Design review of the part built by this model. Coordinates are the model's own, in mm. Coordinates: 2 decimals unless noted, no trailing zeros. Write each loop counter-clockwise with the first axis right and the second up, starting at its lowest first coordinate (ties: lowest second). Pieces come first, ordered by that corner, then holes. Notation, with made-up numbers: (18, 20) - (28, 20) arc R20 ccw to (28, 53) - close; hole circle Ø11 at (-1.75, 51.5). An arc over 180 degrees is marked (long way). Answer as a JSON object with one key per item and string values.
Autodesk Inventor part; units mm, degrees
ref_plane "YZ Plane" through (0, 0, 0) normal (1, 0, 0) x (0, 1, 0)
ref_plane "XZ Plane" through (0, 0, 0) normal (0, 1, 0) x (-1, 0, 0)
ref_plane "XY Plane" through (0, 0, 0) normal (0, 0, 1) x (1, 0, 0)
sketch "Boceto1" plane through (0, 0, 0) normal (0, 0, 1) x (1, 0, 0)
  line L0 (0, 0) -> (220, 0)
  line L1 (251, 0) -> (251, -25)
  line L2 (251, -25) -> (0, -25)
  line L3 (220, 0) -> (220, 85)
  line L4 (220, 85) -> (251, 85)
  line L5 (251, 85) -> (251, 0)
  line L6 (0, -25) -> (-30, -25)
  line L7 (-30, -25) -> (-30, 0)
  line L8 (-30, 0) -> (0, 0)
  dimension "d3" = 85
  dimension "d4" = 31
extrude "Extrusión1" add sketch "Boceto1" along normal blind 10
fillet "Empalme1" radius 30 1 edges at (220, 0, 5)
sketch "Boceto2" plane through (0, 0, 10) normal (0, 0, 1) x (1, 0, 0)
  line L0 (220, 30) -> (220, 85)
  line L1 (251, -25) -> (-30, -25)
  line L2 (220, 85) -> (251, 85)
  line L3 (225.1, 75) -> (239.9, 75)
  line L4 (239.9, 75) -> (239.9, 46)
  line L5 (239.9, 46) -> (225.1, 46)
  line L6 (225.1, 46) -> (225.1, 75)
  line L7 (225.1, 14) -> (239.9, 14)
  line L8 (239.9, 14) -> (239.9, -15)
  line L9 (239.9, -15) -> (225.1, -15)
  line L10 (225.1, -15) -> (225.1, 14)
  point P0 (225, 80)
  point P1 (220, 75)
  point P2 (5, -25)
  point P3 (240, -25)
  point P4 (245, -20)
  point P5 (245, 75)
  point P6 (240, 80)
  point P7 (0, 0)
  point P8 (0, -25)
  dimension "d10" = 14.8
  dimension "d11" = 14.8
  dimension "d12" = 5.1
  dimension "d14" = 10
  dimension "d15" = 29
  dimension "d16" = 29
  dimension "d17" = 10
  dimension "d82" = 5.1
extrude "Extrusión2" cut sketch "Boceto2" against normal blind 10
sketch "Boceto3" plane through (0, 0, 10) normal (0, 0, 1) x (1, 0, 0)
  line L0 (0, 0) -> (190, 0)
  line L1 (251, -25) -> (-30, -25)
  line L2 (180, -10) -> (170, -10)
  line L3 (170, -10) -> (170, -5)
  line L4 (170, -5) -> (180, -5)
  line L5 (180, -5) -> (180, -10)
  line L6 (110, -5) -> (100, -5)
  line L7 (100, -5) -> (100, -10)
  line L8 (100, -10) -> (110, -10)
  line L9 (110, -10) -> (110, -5)
  line L10 (40, -5) -> (30, -5)
  line L11 (30, -5) -> (30, -10)
  line L12 (30, -10) -> (40, -10)
  line L13 (40, -10) -> (40, -5)
  line L14 (145, -15) -> (135, -15)
  line L15 (135, -15) -> (135, -20)
  line L16 (135, -20) -> (145, -20)
  line L17 (145, -20) -> (145, -15)
  line L18 (75, -15) -> (65, -15)
  line L19 (65, -15) -> (65, -20)
  line L20 (65, -20) -> (75, -20)
  line L21 (75, -20) -> (75, -15)
  point P0 (5, 0)
  point P1 (0, -5)
  point P2 (0, -20)
  point P3 (5, -25)
  point P4 (240, -25)
  dimension "d20" = 10
  dimension "d21" = 10
  dimension "d22" = 10
  dimension "d24" = 5
  dimension "d25" = 5
  dimension "d26" = 5
  dimension "d27" = 5
  dimension "d28" = 5
  dimension "d29" = 10
  dimension "d30" = 10
  dimension "d31" = 5
  dimension "d32" = 5
  dimension "d33" = 5
  dimension "d34" = 5
  dimension "d36" = 25
  dimension "d37" = 25
  dimension "d38" = 25
  dimension "d39" = 25
extrude "Extrusión3" cut sketch "Boceto3" against normal blind 10
sketch "Boceto4" plane through (0, 0, 10) normal (0, 0, 1) x (1, 0, 0)
  line L0 (145, -15) -> (145, -20)
  line L1 (145, -20) -> (135, -20)
  line L2 (205, -20) -> (215, -20)
  line L3 (215, -20) -> (215, -15)
  line L4 (215, -15) -> (205, -15)
  line L5 (205, -15) -> (205, -20)
  point P0 (0, 0)
  dimension "d42" = 10
  dimension "d43" = 5
  dimension "d44" = 60
extrude "Extrusión4" cut sketch "Boceto4" against normal blind 10
sketch "Boceto6" plane through (0, 0, 10) normal (0, 0, 1) x (1, 0, 0)
  line L0 (237.5, 82.5) -> (227.5, 82.5)
  line L1 (227.5, 82.5) -> (227.5, 77.5)
  line L2 (227.5, 77.5) -> (237.5, 77.5)
  line L3 (237.5, 77.5) -> (237.5, 82.5)
  circle A0 centre (245.5, -17.5) radius 1.6
  circle A1 centre (245.5, 27.5) radius 1.6
  circle A2 centre (245.5, 75.9891) radius 1.6
  circle A3 centre (222.4918, 80) radius 1.6
  circle A4 centre (222.4918, 27.5) radius 1.6
  circle A5 centre (175, -17.5) radius 1.6
  circle A6 centre (166.25, -7.5) radius 1.6
  circle A7 centre (105, -17.5) radius 1.6
  circle A8 centre (70, -7.5) radius 1.6
  circle A9 centre (45, -17.5) radius 1.6
  circle A10 centre (0, -7.5) radius 1.6
  line L4 (-30, -25) -> (-30, 0)
  circle A11 centre (222.4918, -17.5) radius 1.6
  line L5 (251, 85) -> (251, -25)
  line L6 (220, 85) -> (251, 85)
  line L7 (170, -10) -> (170, -5)
  point P0 (0, 0)
  dimension "d52" = 5
  dimension "d54" = 3.2
  dimension "d55" = 3.2
  dimension "d56" = 3.2
  dimension "d57" = 3.2
  dimension "d58" = 3.2
  dimension "d60" = 3.2
  dimension "d61" = 3.2
  dimension "d62" = 3.2
  dimension "d63" = 3.2
  dimension "d64" = 3.2
  dimension "d65" = 3.2
  dimension "d80" = 30
  dimension "d81" = 3.2
  dimension "d83" = 5.5
  dimension "d84" = 5.5
  dimension "d85" = 5.5
  dimension "d92" = 2.5
  dimension "d93" = 5
  dimension "d94" = 3.75
  dimension "d95" = 75
extrude "Extrusión6" cut sketch "Boceto6" against normal blind 10
fillet "Empalme3" radius 5 1 edges at (251, -25, 5)
fillet "Empalme4" radius 5 2 edges at (-30, 0, 5) (-30, -25, 5)
fillet "Empalme5" radius 1 2 edges at (220, 85, 5) (251, 85, 5)
sketch "Boceto7" plane through (0, 0, 10) normal (0, 0, 1) x (1, 0, 0)
  line L0 (-25, 0) -> (190, 0)
  line L1 (-30, -20) -> (-30, -5)
  line L2 (-25, -5) -> (-15, -5)
  line L3 (-15, -5) -> (-15, -20)
  line L4 (-15, -20) -> (-25, -20)
  line L5 (-25, -20) -> (-25, -5)
  point P0 (0, 0)
  dimension "d74" = 10
  dimension "d75" = 15
  dimension "d76" = 5
  dimension "d77" = 5
extrude "Extrusión7" cut sketch "Boceto7" against normal blind 10
sketch "Boceto8" plane through (0, 0, 10) normal (0, 0, 1) x (1, 0, 0)
  line L0 (221, 85) -> (250, 85)
  line L1 (251, 84) -> (251, -20)
  line L2 (243, 66.5) -> (248, 66.5)
  line L3 (248, 66.5) -> (248, 56.5)
  line L4 (248, 56.5) -> (243, 56.5)
  line L5 (243, 56.5) -> (243, 66.5)
  point P0 (0, 0)
  dimension "d86" = 5
  dimension "d87" = 10
  dimension "d88" = 3
  dimension "d89" = 18.5
extrude "Extrusión8" cut sketch "Boceto8" against normal blind 10
properties part number "brazo eje z"
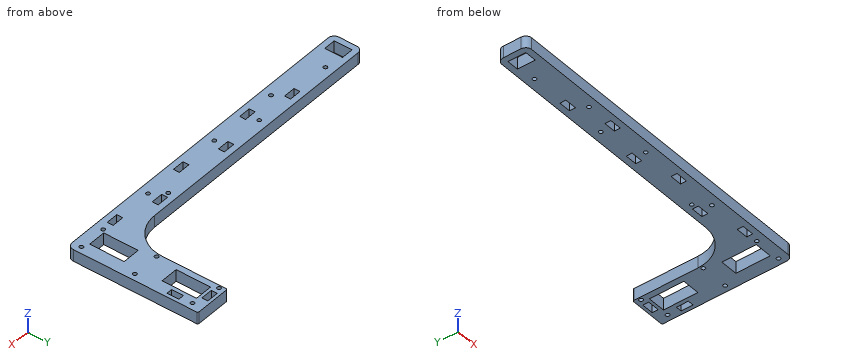
(1) Take a section at B-B, the plane x = 18.5. Write out the cut boundary in (y, z), and give its area (3 significant figures).
Solved:
{"outline": "(-25, 0) - (0, 0) - (0, 10) - (-25, 10) - close", "area": "250 mm^2"}
(2) Take a section at A-A, the plane y = 6. Write out the cut boundary in (x, z).
Solved:
{"outline": "(208, 0) - (225.1, 0) - (225.1, 10) - (208, 10) - close; (239.9, 0) - (251, 0) - (251, 10) - (239.9, 10) - close"}
(3) For pin 1 (10 mm diameter, centred on x = 3, y = -9.5, fed in from -Z); pin 2 (1.5 mm diameter, centred on y = 70, z = 2.5, fed in from -X); pin 3 (6 mm diameter, centred on y = 24, z = 8.5, fed in from -X), all flat-tipped, find the tip position at first contact; note any pin that passes through.
Solved:
{"pin 1": "stops at z = 0", "pin 2": "stops at x = 220", "pin 3": "stops at x = 218.62"}
(4) Take a section at C-C, the plane z = 3. Give the number of separate pieces and of enclosed holes in the cut face, and give its area (3 significant figures).
Solved:
{"separate pieces": "1", "enclosed holes": "23", "area": "8,330 mm^2"}
(5) To check wall thickness, follow line 1 (X direction, y = 80, z = 7.5); line 2 (Y direction, x = 175, z = 4); line 3 (X direction, y = 64, z = 6). State the ranges of each line that lie inside material, in increasing order. Write a range as from..to.
Solved:
{"line 1": "x = 220..220.89, 224.09..227.5, 237.5..251", "line 2": "y = -25..-19.1, -15.9..-10, -5..0", "line 3": "x = 220..225.1, 239.9..243, 248..251"}
